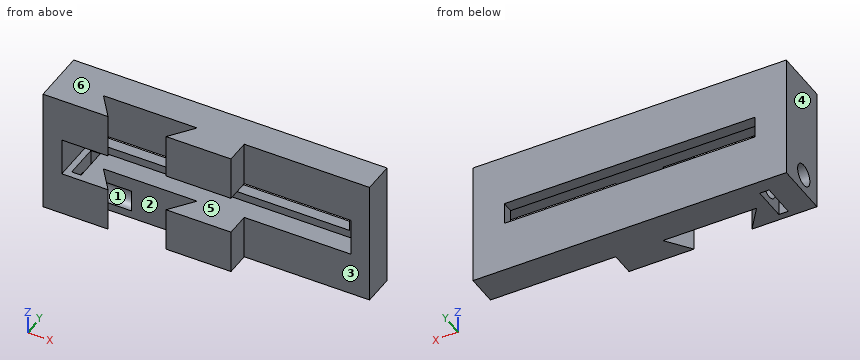
```python
from build123d import *

# Parameters (mm, degrees)
F0_W      = 50
F0_H      = 20
F1_DEPTH  = 5
F2_W      = 30
F2_H      = 20
F3_DEPTH  = 3.8
F4_W      = 15.25
F4_H      = 20
F5_DEPTH  = 4
F6_SIZE2  = 3.99999
F6_SIZE   = 2.99999
F9_W      = 40
F9_H      = 3.5
F10_DEPTH = 12.5
F11_W     = 44
F11_H     = 6
F12_DEPTH = 7
F13_R     = 1.75
F14_DEPTH = 12
F15_W     = 1.5
F15_H     = 5.5
F16_DEPTH = 8


# Not quite as in the source:
# - a fillet or chamfer is up to 0.001 mm smaller than in the source, because OpenCascade refuses the exact size


with BuildPart() as f1:
    # F0 (on Front) → F1 (new body)
    with BuildSketch(Plane.XZ):
        Rectangle(F0_W, F0_H)
    extrude(amount=F1_DEPTH)


with BuildPart() as f3:
    # F2 (on face) → F3 (new body)
    with BuildSketch(Plane.XZ.offset(5)):
        with Locations((-10, 0)):
            Rectangle(F2_W, F2_H)
    extrude(amount=F3_DEPTH)


with BuildPart() as f5:
    # F4 (on face) → F5 (new body)
    with BuildSketch(Plane.XZ.offset(8.8)):
        with Locations((-9.995, 0)):
            Rectangle(F4_W, F4_H)
    extrude(amount=-F5_DEPTH)

    # F6 (size 3 and 4 in the source; OpenCascade refuses exactly that, so slightly less here)
    f6_edges = [f5.edges().sort_by_distance(p)[0] for p in [
        (-2.37, -8.8, 0),
        (-17.62, -8.8, 0),
    ]]
    f6_side = f5.faces().sort_by_distance((-9.995, -8.8, 0))[0]
    chamfer(f6_edges, length=F6_SIZE, length2=F6_SIZE2, reference=f6_side)


with BuildPart() as f3_1:
    add(f3.part)

    # F7: cut F5
    add(f5.part, mode=Mode.SUBTRACT)


with BuildPart() as f1_1:
    add(f1.part)

    # F8: union F3
    add(f3_1.part)

    # F9 (on face) → F10 (cut, symmetric)
    with BuildSketch(Plane.XZ.offset(8.8)):
        Rectangle(F9_W, F9_H)
    extrude(amount=F10_DEPTH, both=True, mode=Mode.SUBTRACT)

    # F11 (on face) → F12 (cut)
    with BuildSketch(Plane.XZ.offset(8.8)):
        Rectangle(F11_W, F11_H)
    extrude(amount=-F12_DEPTH, mode=Mode.SUBTRACT)

    # F13 (on face) → F14 (cut)
    with BuildSketch(Plane(origin=(-25, 0, 0), x_dir=(0, -1, 0), z_dir=(-1, 0, 0))):
        with Locations((5, -7)):
            Circle(F13_R)
    extrude(amount=-F14_DEPTH, mode=Mode.SUBTRACT)

    # F15 (on face) → F16 (cut)
    with BuildSketch(Plane(origin=(0, 0, -10), x_dir=(1, 0, 0), z_dir=(0, 0, -1))):
        with Locations((-20.25, 5)):
            Rectangle(F15_W, F15_H)
    extrude(amount=-F16_DEPTH, mode=Mode.SUBTRACT)


solid = f1_1.part
```
Source: CAD feature listing. Evaluate the final solid. Frame: model axes, mm. Face numbers are marked on the shaded views. A direction names the side the tool comes from. Coordinates: 2 decimals unless noted, no trailing zeros. Loops run counter-clockwise (first coordinate to the right, second up) from the corner with the lowest first, then second, coordinate; pieces in that order, holes last. Notation, with made-up numbers: (10, 87) - (50, 87) arc R20 ccw to (50, 107) - close; hole circle Ø4 at (-24.5, 4). An arc over 180 degrees is marked (long way). Answer as CSV lines item,"result".
1. Section C-C (z = -4.5). Return loops of the section in (x, y), then the cut area to 3 significant figures.
Established:
outline,"(-25, -8.8) - (-14.62, -8.8) - (-17.47, -5) - (-2.52, -5) - (-5.37, -8.8) - (5, -8.8) - (5, -5) - (25, -5) - (25, 0) - (-25, 0) - close; hole (-21, -7.75) - (-19.5, -7.75) - (-19.5, -2.25) - (-21, -2.25) - close"
area,"310 mm2"
2. Section D-D (z = -1.25). Return loops of the section in (x, y), then the cut area to 3 significant figures.
Established:
outline,"(-25, -8.8) - (-22, -8.8) - (-22, -1.8) - (-20, -1.8) - (-20, 0) - (-25, 0) - close; (20, -1.8) - (22, -1.8) - (22, -5) - (25, -5) - (25, 0) - (20, 0) - close"
area,"48.6 mm2"
3. Ray query, line 1 (Z direction, x = -17.5, y = -5); line 2 (Z direction, x = 15, y = -3.5); line 3 (Y direction, x = -16.5, z = -7). Return the intervals inside material, ascending.
Established:
line 1,"z = -10 to -8.75, -5.25 to -3, 3 to 10"
line 2,"z = -10 to -3, 3 to 10"
line 3,"y = -8.8 to -6.75, -3.25 to 0"
4. Reachability of the marked faces 1, 2 and 3 from +Z, -Z, +X, -X, +Y, -Y: full face, straight path, thin tool, end or side. Return the list, or none.
Established:
face 1,"-X"
face 2,"+Z, -Z"
face 3,"+Z, -Z, +X, -Y"
5. Mould query, pull axis X, two halves, no side actions, for the marked faces 4, 5 and 6. Classes: released by +X, released by -X, zero draft, split by the parting line, or undercut.
Established:
face 4,"released by -X"
face 5,"undercut"
face 6,"zero draft"
6. Section A-A (x = 1). Return loops of the section in (y, z).
Established:
outline,"(-8.8, -10) - (0, -10) - (0, -1.75) - (-1.8, -1.75) - (-1.8, -3) - (-8.8, -3) - close; (-8.8, 3) - (-1.8, 3) - (-1.8, 1.75) - (0, 1.75) - (0, 10) - (-8.8, 10) - close"
7. Contact query for flat-ended pins moving along their axis: pin 1 (4 mm diameter, centred on y = -5, z = -7, fed in from -X); pin 2 (3 mm diameter, centred on y = -7, z = 7.5, fed in from +X); pin 3 (3.5 mm diameter, centred on x = -9.5, z = -5, fed in from -Y). Output: stop coordinate, or through.
Established:
pin 1,"stops at x = -25"
pin 2,"stops at x = 5"
pin 3,"stops at y = -5"
8. Section B-B (y = -1). Return loops of the section in (x, z).
Established:
outline,"(-25, -10) - (25, -10) - (25, 10) - (-25, 10) - close; hole (-20, -1.75) - (20, -1.75) - (20, 1.75) - (-20, 1.75) - close"
